```python
from build123d import *

# Parameters (mm, degrees)
BOSS_EXTRUDE1_DEPTH  = 7
M3_CLEARANCE_HOLE1_D = 3.2
CHAMFER2_SIZE        = 0.25
FILLET1_R            = 1


with BuildPart() as part:
    # Sketch1 → Boss-Extrude1 (new body)
    with BuildSketch(Plane(origin=(0, 0, 0), x_dir=(1, 0, 0), z_dir=(0, 1, 0))):
        with BuildLine():
            Line((0, 0), (-5, 0))
            Line((-5, 0), (-5, 9))
            Line((-5, 9), (-5, 15))
            ThreePointArc((-5, 15), (-3.828427125, 17.828427125), (-1, 19))
            Line((-1, 19), (0, 19))
            Line((0, 19), (0, 17))
            Line((0, 17), (-1, 17))
            ThreePointArc((-1, 17), (-3, 15), (-1, 13))
            Line((-1, 13), (0, 13))
            Line((0, 13), (0, 11))
            Line((0, 11), (-1, 11))
            ThreePointArc((-1, 11), (-3, 9), (-1, 7))
            Line((-1, 7), (0, 7))
            Line((0, 7), (0, 0))
        make_face()
    extrude(amount=BOSS_EXTRUDE1_DEPTH)

    # M3 Clearance Hole1 (through all)
    with Locations(Plane.ZY.offset(5)):
        with Locations((-3.5, 3.5)):
            Hole(M3_CLEARANCE_HOLE1_D / 2)

    # Chamfer2
    chamfer2_edges = [part.edges().sort_by_distance(p)[0] for p in [
        (-5, 3.5, -1.9),
        (0, 3.5, -1.9),
    ]]
    chamfer(chamfer2_edges, length=CHAMFER2_SIZE)

    # Fillet1
    fillet1_edges = [part.edges().sort_by_distance(p)[0] for p in [
        (-5, 3.5, 0),
    ]]
    fillet(fillet1_edges, radius=FILLET1_R)


solid = part.part
```
Model file for the job. Use its own axes, mm. A direction names the side the tool comes from. Coordinates: 2 decimals unless noted, no trailing zeros. Order: outer loops, then holes, each group sorted by start corner. A loop starts at its lowest first (then second) coordinate and runs counter-clockwise, first axis right, second up. Notation, with made-up numbers: (-32.5, 27.5) - (-7.5, 27.5) arc R15 cw to (-7.5, 47.5) - close; hole circle Ø4 at (76.25, 74). An arc over 180 degrees is marked (long way). Return JSON: item names as keys, results as strings. Group by question number.
1) Saw through at A-A, the plane z = -3.5. Write the cut outline in (x, y), plus the area to 3 significant figures.
2) Probe line 1 (Z direction, x = -0.45, y = 6.75); line 2 (Y direction, x = -1.5, z = -3.5); line 3 (Z direction, x = -2.55, y = 4.75). List the from-to ranges inside material, lowest first. Write a range as from..to.
3) Tool access for faces 1 (the flat face through (-0.5, 3.5, -17)), 2 (the flat face through (0, 3, -18)): list every direction of +Z, -Z, +X, -X, +Y, -Y with a clear straight run to the whole face (end or side of a thin tool).
4) Saw through at B-B, the plane x = -2.45. Write the cut outline in (y, z).
5) Saw through at C-C, the plane x = -3.8. Write the cut outline in (y, z), plus the area to 3 significant figures.
6) Mould opens along Z. For faces 3 (the cylindrical face through (-3, 3, -9)), 4 (the flat face through (-3, 7, -8)), 5 (the cylindrical face through (-3.859, 3.451, -17.797)), 6 (the flat face through (-2, 3, 0)) say: released by +Z, released by -Z, zero draft, split by the parting line, or undercut.
7) Flat gauge pin, fed straight in: P1, Ø3, axis at x = -1.5, y = 6, coming from the -Z side. Where does the tip first touch, or does it go through?
8) Saw through at D-D, the plane x = -1.6. Write the cut outline in (y, z).
Values found:
{
 "1": {"outline": "(-5, 0) - (0, 0) - (0, 1.65) - (-0.25, 1.9) - (-4.75, 1.9) - (-5, 1.65) - close; (-5, 5.35) - (-4.75, 5.1) - (-0.25, 5.1) - (0, 5.35) - (0, 7) - (-5, 7) - close", "area": "18.9 mm²"},
 "2": {"line 1": "z = -19..-17, -13..-11, -7..0", "line 2": "y = 0..1.9, 5.1..7", "line 3": "z = -18.69..-16.26, -13.74..-10.26, -7.74..-4.5, -2.5..0"},
 "3": {"face 1": "+X, +Y, -Y", "face 2": "+Z, -Z, +X, +Y, -Y"},
 "4": {"outline": "(0, -18.73) - (7, -18.73) - (7, -16.38) - (0, -16.38) - close; (0, -13.62) - (7, -13.62) - (7, -10.38) - (0, -10.38) - close; (0, -7.62) - (7, -7.62) - (7, 0) - (0, 0) - close; hole circle Ø3.2 at (3.5, -3.5)"},
 "5": {"outline": "(0, -17.86) - (7, -17.86) - (7, 0) - (0, 0) - close; hole circle Ø3.2 at (3.5, -3.5)", "area": "117 mm²"},
 "6": {"face 3": "undercut", "face 4": "zero draft", "face 5": "released by -Z", "face 6": "released by +Z"},
 "7": {"P1": "stops at z = -19"},
 "8": {"outline": "(0, -18.95) - (7, -18.95) - (7, -16.91) - (0, -16.91) - close; (0, -13.09) - (7, -13.09) - (7, -10.91) - (0, -10.91) - close; (0, -7.09) - (7, -7.09) - (7, 0) - (0, 0) - close; hole circle Ø3.2 at (3.5, -3.5)"}
}
